Part model, mm, in its own coordinate system. Give positions to 0.01 mm unless a question says otherwise; leave off trailing zeros. Write each loop counter-clockwise with the first axis right and the second up, starting at its lowest first coordinate (ties: lowest second). Pieces come first, ordered by that corner, then holes. Notation, with made-up numbers: M 44,-1 L 82,-1 A15 cw 82,16 Z; hole C 22,86.5 d11. An arc over 180 degrees is marked long. Use CSV: the item, a comma, the result in double quotes. Start each with the question number.
1. Drill centre lines: line 1 along Z through (x, y) = (3.5, -34); line 2 along Y through (x, z) = (-1, 1.5); line 3 along Y through (x, z) = (-2.25, 6.5). Where is each one in solid material? Low to high. Write a range as from..to.
2. Mould opens along Y. For faces 1 (the face through (4, 1, 5.08)), 2 (the face through (-2, 1, 0)) say: pulls with the +Y half, pulls with the -Y half, needs draft (parallel to the pull), parting line crosses it, or undercut.
3. Band-saw the part on B-B, the plane x = 2.75. List the corners of the cut face in (y, z) (3 decimals), then the cut area to 3 significant figures.
4. Band-saw the part on C-C, the plane y = 15. List the corners of the cut face in (x, z), then the cut area to 3 significant figures.
5. Drop flat-ended pins along their axis: pin 1 Ø3 at (x, y) = (2.5, 27.5) entering from +Z; pin 2 Ø2 at (x, z) = (-2.5, 7) entering from -Y; pin 3 Ø4 at (x, y) = (0, -34.925) entering from +Z (3 decimals). Give the stop position or say it passes through.
6. Band-saw the part on A-A, the plane z = 6.25. List the corners of the cut face in (x, y) (1 decimal), then the cut area to 3 significant figures.
from build123d import *

# Parameters (mm, degrees)
F1_DEPTH = 5.08
F2_DEPTH = 9.525


with BuildPart() as f1:
    # F0 (on Top) → F1 (new body)
    with BuildSketch(Plane.XY):
        with BuildLine():
            ThreePointArc((0, -41.275), (4.4901280605, -39.4151280605), (6.35, -34.925))
            Line((6.35, -34.925), (6.35, 34.925))
            ThreePointArc((6.35, 34.925), (4.4901280605, 39.4151280605), (0, 41.275))
            ThreePointArc((0, 41.275), (-4.4901280605, 39.4151280605), (-6.35, 34.925))
            Line((-6.35, 34.925), (-6.35, -34.925))
            ThreePointArc((-6.35, -34.925), (-4.4901280605, -39.4151280605), (0, -41.275))
        make_face()
        with BuildLine():
            ThreePointArc((3.4925, -34.925), (-2.4695704333, -37.3945704333), (0, -31.4325))
            ThreePointArc((0, -31.4325), (2.4695704333, -32.4554295667), (3.4925, -34.925))
        make_face(mode=Mode.SUBTRACT)
        with BuildLine():
            ThreePointArc((0, -27.305), (-1.905, -25.4), (0, -23.495))
            ThreePointArc((0, -23.495), (1.3470384182, -24.0529615818), (1.905, -25.4))
            ThreePointArc((1.905, -25.4), (1.3470384182, -26.7470384182), (0, -27.305))
        make_face(mode=Mode.SUBTRACT)
        with BuildLine():
            ThreePointArc((0, -3.4925), (-3.4925, 0), (0, 3.4925))
            ThreePointArc((0, 3.4925), (2.4695704333, 2.4695704333), (3.4925, 0))
            ThreePointArc((3.4925, 0), (2.4695704333, -2.4695704333), (0, -3.4925))
        make_face(mode=Mode.SUBTRACT)
        with BuildLine():
            ThreePointArc((0, 23.495), (-1.905, 25.4), (0, 27.305))
            ThreePointArc((0, 27.305), (1.3470384182, 26.7470384182), (1.905, 25.4))
            ThreePointArc((1.905, 25.4), (1.3470384182, 24.0529615818), (0, 23.495))
        make_face(mode=Mode.SUBTRACT)
        with BuildLine():
            ThreePointArc((3.4925, 34.925), (2.4695704333, 32.4554295667), (0, 31.4325))
            ThreePointArc((0, 31.4325), (-2.4695704333, 37.3945704333), (3.4925, 34.925))
        make_face(mode=Mode.SUBTRACT)
    extrude(amount=F1_DEPTH)

    # F0 (on Top) → F2 (join)
    with BuildSketch(Plane.XY):
        with BuildLine():
            ThreePointArc((3.4925, -34.925), (2.4695704333, -32.4554295667), (0, -31.4325))
            ThreePointArc((0, -31.4325), (-2.4695704333, -37.3945704333), (3.4925, -34.925))
        make_face()
        with BuildLine():
            ThreePointArc((1.4605, -34.925), (-1.0327294539, -35.9577294539), (0, -33.4645))
            ThreePointArc((0, -33.4645), (1.0327294539, -33.8922705461), (1.4605, -34.925))
        make_face(mode=Mode.SUBTRACT)
        with BuildLine():
            ThreePointArc((3.4925, 0), (2.4695704333, 2.4695704333), (0, 3.4925))
            Line((0, 3.4925), (0, 1.4605))
            ThreePointArc((0, 1.4605), (1.0327294539, 1.0327294539), (1.4605, 0))
            ThreePointArc((1.4605, 0), (1.0327294539, -1.0327294539), (0, -1.4605))
            Line((0, -1.4605), (0, -3.4925))
            ThreePointArc((0, -3.4925), (2.4695704333, -2.4695704333), (3.4925, 0))
        make_face()
        with BuildLine():
            Line((0, 1.4605), (0, 3.4925))
            ThreePointArc((0, 3.4925), (-3.4925, 0), (0, -3.4925))
            Line((0, -3.4925), (0, -1.4605))
            ThreePointArc((0, -1.4605), (-1.4605, 0), (0, 1.4605))
        make_face()
        with BuildLine():
            ThreePointArc((3.4925, 34.925), (-2.4695704333, 37.3945704333), (0, 31.4325))
            ThreePointArc((0, 31.4325), (2.4695704333, 32.4554295667), (3.4925, 34.925))
        make_face()
        with BuildLine():
            ThreePointArc((1.4605, 34.925), (1.0327294539, 33.8922705461), (0, 33.4645))
            ThreePointArc((0, 33.4645), (-1.0327294539, 35.9577294539), (1.4605, 34.925))
        make_face(mode=Mode.SUBTRACT)
    extrude(amount=F2_DEPTH)


solid = f1.part
Output:
1,line 1,"z = 0..5.08"
1,line 2,"y = -41.2..-35.99, -33.86..-27.02, -23.78..-1.06, 1.06..23.78, 27.02..33.86, 35.99..41.2"
1,line 3,"y = -37.6..-32.25, -2.67..2.67, 32.25..37.6"
2,face 1,"undercut"
2,face 2,"needs draft"
3,outline,"M -40.649,0 L 40.649,0 L 40.649,5.08 L 37.078,5.08 L 37.078,9.525 L 32.772,9.525 L 32.772,5.08 L 2.153,5.08 L 2.153,9.525 L -2.153,9.525 L -2.153,5.08 L -32.772,5.08 L -32.772,9.525 L -37.078,9.525 L -37.078,5.08 L -40.649,5.08 Z"
3,area,"470 mm²"
4,outline,"M -6.35,0 L 6.35,0 L 6.35,5.08 L -6.35,5.08 Z"
4,area,"64.5 mm²"
5,pin 1,"stops at z = 5.08"
5,pin 2,"stops at y = -38.08"
5,pin 3,"stops at z = 9.525"
6,outline,"C 0,-34.9 d7; C 0,0 d7; C 0,34.9 d7; hole C 0,-34.9 d2.9; hole C 0,0 d2.9; hole C 0,34.9 d2.9"
6,area,"94.9 mm²"
